CAD build for the part. Positions are in the model's coordinates, mm. Round coordinates to 2 decimals unless told otherwise and drop trailing zeros. Loops run counter-clockwise (first coordinate to the right, second up) from the corner with the lowest first, then second, coordinate; pieces in that order, holes last.
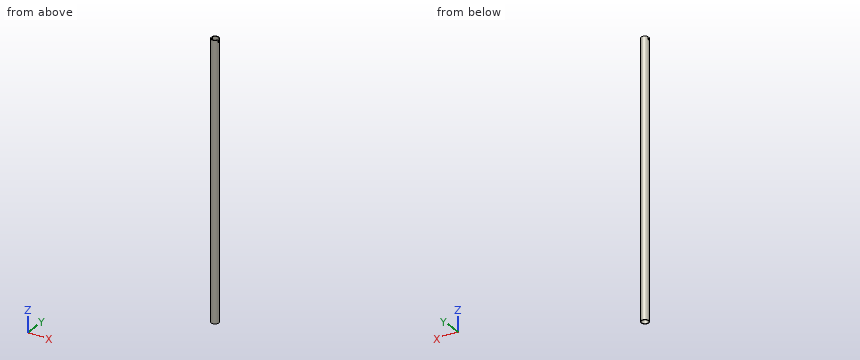
from build123d import *

# Parameters (mm, degrees)
SKETCH4_R           = 33
SKETCH4_R_2         = 29.5
BOSS_EXTRUDE1_DEPTH = 2380
CUT_EXTRUDE1_DEPTH  = 67
FILLET1_R           = 1


with BuildPart() as part:
    # Sketch4 → Boss-Extrude1 (new body)
    with BuildSketch(Plane.XY):
        with Locations((33, 0)):
            Circle(SKETCH4_R)
        with Locations((33, 0)):
            Circle(SKETCH4_R_2, mode=Mode.SUBTRACT)
    extrude(amount=-BOSS_EXTRUDE1_DEPTH)

    # Sketch6 → Cut-Extrude1 (cut, through all)
    with BuildSketch(Plane(origin=(0, 0, 0), x_dir=(0, 0, -1), z_dir=(1, 0, 0))):
        with BuildLine():
            Line((0, 10), (0, -10))
            Line((0, -10), (15, -10))
            ThreePointArc((15, -10), (25, 0), (15, 10))
            Line((15, 10), (0, 10))
        make_face()
    extrude(amount=CUT_EXTRUDE1_DEPTH, mode=Mode.SUBTRACT)

    # Fillet1
    fillet1_edges = [part.edges().sort_by_distance(p)[0] for p in [
        (3.39912572, 10, 0),
        (62.60087428, 10, 0),
        (3.39912572, -10, 0),
        (62.60087428, -10, 0),
    ]]
    fillet(fillet1_edges, radius=FILLET1_R)


solid = part.part
Item 1: Cut at B-B (x = 33). List the corners of the cut face in (y, z), plus the area to 3 significant figures.
Verdict:
outline: (-33, -2380) - (-29.5, -2380) - (-29.5, 0) - (-33, 0) - close; (29.5, -2380) - (33, -2380) - (33, 0) - (29.5, 0) - close
area: 16,700 mm2
Item 2: Cut at A-A (y = 0). List the corners of the cut face in (x, z).
Verdict:
outline: (0, -2380) - (3.5, -2380) - (3.5, -25) - (0, -25) - close; (62.5, -2380) - (66, -2380) - (66, -25) - (62.5, -25) - close
Item 3: Flat gauge pins, fed straight in: P1, Ø4, axis at x = 21, z = -679, coming from the -Y side; P2, Ø3, axis at x = 63, z = -10, coming from the +Y side; P3, Ø5, axis at x = 31, z = -482, coming from the +Y side; P4, Ø1, axis at x = 57, y = -21.5, coming from the +Z side. Where does each tip first touch, or does it go through?
Verdict:
P1: stops at y = -31.45
P2: stops at y = 16.64
P3: stops at y = 33
P4: stops at z = 0
Item 4: Wall check: L1, parallel to Y at x = 35, z = -1099; L2, parallel to X at y = 0, z = -1620.5; L3, parallel to Y at x = 33, z = -1719. Give the ranges that are in metal, low to high.
Verdict:
L1: y = -32.94 to -29.43, 29.43 to 32.94
L2: x = 0 to 3.5, 62.5 to 66
L3: y = -33 to -29.5, 29.5 to 33
Item 5: Cut at C-C (z = -2153). List the corners of the cut face in (x, y).
Verdict:
outline: circle Ø66 at (33, 0); hole circle Ø59 at (33, 0)
